from build123d import *

# Parameters (mm, degrees)
F0_W     = 86
F0_H     = 55
F1_DEPTH = 5
F2_W     = 80.4
F2_H     = 49.4
F3_DEPTH = 2
F4_R     = 2


with BuildPart() as f1:
    # F0 (on Top) → F1 (new body)
    with BuildSketch(Plane.XY):
        Rectangle(F0_W, F0_H)
    extrude(amount=F1_DEPTH)

    # F2 (on face) → F3 (join)
    with BuildSketch(Plane.XY.offset(5)):
        with Locations((-0.2, 0.2)):
            Rectangle(F2_W, F2_H)
    extrude(amount=F3_DEPTH)

    # F4
    f4_edges = [f1.edges().sort_by_distance(p)[0] for p in [
        (-40.4, -24.5, 6),
        (-40.4, 24.9, 6),
        (40, -24.5, 6),
        (40, 24.9, 6),
    ]]
    fillet(f4_edges, radius=F4_R)


solid = f1.part
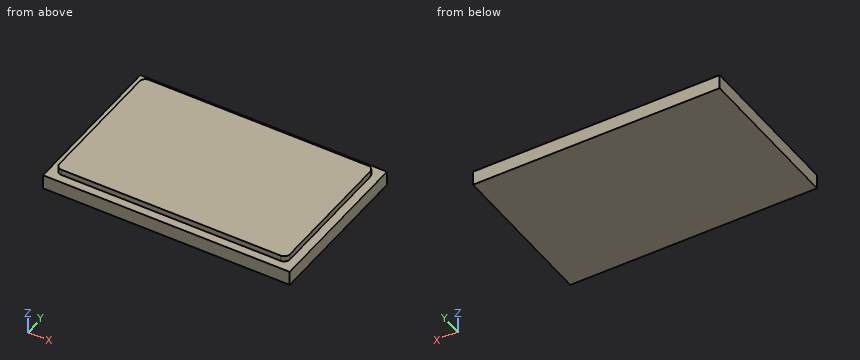
Here's how the part is built. I have some questions about the finished solid (model axes, mm). Coordinates: 2 decimals unless noted, no trailing zeros. Order: outer loops, then holes, each group sorted by start corner. A loop starts at its lowest first (then second) coordinate and runs counter-clockwise, first axis right, second up.
Item 1: I need wall thicknesses on line 1 (X direction, y = 15, z = 5.5); line 2 (Y direction, x = 27.5, z = 6.5); line 3 (X direction, y = 24, z = 6.75). Which ranges of each line are inside material? Lowest first, please.
Result sheet:
line 1: x = -40.4 to 40
line 2: y = -24.5 to 24.9
line 3: x = -40.07 to 39.67
Item 2: If we section it at A-A on y = 18: List the corners of the cut face in (x, z) for me, plus the area to 3 significant figures.
Result sheet:
outline: (-43, 0) - (43, 0) - (43, 5) - (40, 5) - (40, 7) - (-40.4, 7) - (-40.4, 5) - (-43, 5) - close
area: 591 mm2
Item 3: If we section it at B-B on x = 11: List the corners of the cut face in (y, z) for me.
Result sheet:
outline: (-27.5, 0) - (27.5, 0) - (27.5, 5) - (24.9, 5) - (24.9, 7) - (-24.5, 7) - (-24.5, 5) - (-27.5, 5) - close
Item 4: For P1, Ø0.6, axis at x = -15.5, z = 6.5, coming from the +Y side; P2, Ø0.6, axis at x = -13, z = 5.5, coming from the -Y side; P3, Ø0.6, axis at y = 7.5, z = 6, coming from the +X side, each with a flat end and sliding along its axis, tell me the tip position at first contact or that it passes through.
Result sheet:
P1: stops at y = 24.9
P2: stops at y = -24.5
P3: stops at x = 40
